Can you work these out from the model? Positions are in its coordinate system, mm. A direction names the side the tool comes from. Coordinates: 2 decimals unless noted, no trailing zeros. Order: outer loops, then holes, each group sorted by start corner. A loop starts at its lowest first (then second) coordinate and runs counter-clockwise, first axis right, second up. Notation, with made-up numbers: (63.5, 5) - (67.5, 5) arc R29 ccw to (67.5, 29) - close; hole circle Ø2 at (20, 35). An arc over 180 degrees is marked (long way). Return JSON: item names as keys, results as strings. Group by question number.
1) Imagine slicing it at C-C (z = -1). Give the number of separate pieces and of enclosed holes in the cut face, and give its area (3 significant figures).
2) Which directions (+Z, -Z, +X, -X, +Y, -Y) give clear straight access to the entire face, cutting with the end or side of a thin tool? Please do faces 4 (the face through (10.377, 0.493, -16.829)), 5 (the face through (-1.235, -2, -6)), 6 (the face through (13, -2, -14.299)), 7 (the face through (2, 7, -7.799)).
3) Imagine slicing it at A-A (z = 2). Write out the boundary of the cut face in (x, y), and give its area (3 significant figures).
4) Imagine slicing it at D-D (x = -13). Write out the boundary of the cut face in (y, z).
5) For pin 1 Ø1.2 at (x, y) = (12.5, -3) entering from -Z; pin 2 Ø0.8 at (x, y) = (-12, 0.5) entering from +Z; pin 3 Ø4 at (x, z) = (-16.5, -16.5) entering from -Y, each with a flat end and sliding along its axis, tell me the tip position at first contact or that it passes through.
6) Imagine slicing it at B-B (x = 25). Write out the boundary of the cut face in (y, z).
7) If we mould it in two halves opening along X, with no side actions, what happens to faces 1 (the face through (13, -5, -7)), 2 (the face through (21, 1, -16)), 3 (the face through (20.765, -2, -6))? For each: pulls with the +X half, pulls with the -X half, needs draft (parallel to the pull), parting line crosses it, or undercut.
8) If I drill on line 1 along X through (y, z) = (8.75, -5.5); line 2 along X through (y, z) = (3, -16.75); line 3 along Z through (x, y) = (-8, 2.75), over which ranges is the centre line in solid material (lowest first)?
```python
from build123d import *

# Parameters (mm, degrees)
SKETCH1_R           = 3
SKETCH1_R_2         = 1.7
BOSS_EXTRUDE1_DEPTH = 1
SKETCH1_4_W         = 1
SKETCH1_4_H         = 0.5
SKETCH1_4_H_2       = 12.5
SKETCH1_4_W_2       = 1.5
SKETCH1_4_W_3       = 2
SKETCH1_4_R         = 1.7
BOSS_EXTRUDE2_DEPTH = 14
SKETCH1_5_W         = 1
SKETCH1_5_H         = 6
SKETCH1_5_H_2       = 0.5
SKETCH1_5_W_2       = 1.5
BOSS_EXTRUDE3_DEPTH = 5


with BuildPart() as part:
    # Sketch1 → Boss-Extrude1 (new body)
    with BuildSketch(Plane(origin=(0, 0, 0), x_dir=(1, 0, 0), z_dir=(0, 1, 0))):
        Polygon((18.764581115, -4.700712669), (40.514581115, -4.700712669), (40.514581115, 20.799287331), (26.264581115, 20.799287331), (26.264581115, 20.299287331), (21.264581115, 20.299287331), (21.264581115, 20.799287331), (11.264581115, 20.799287331), (11.264581115, 20.299287331), (6.264581115, 20.299287331), (6.264581115, 20.799287331), (1.264581115, 20.799287331), (-2.735418885, 20.799287331), (-2.735418885, 20.299287331), (-7.735418885, 20.299287331), (-7.735418885, 20.799287331), (-29.485418885, 20.799287331), (-29.485418885, -4.700712669), (-14.735418885, -4.700712669), (-14.735418885, -4.200712669), (-9.735418885, -4.200712669), (-9.735418885, -4.700712669), (-4.735418885, -4.700712669), (-0.735418885, -4.700712669), (-0.735418885, -4.200712669), (4.264581115, -4.200712669), (4.264581115, -4.700712669), (13.764581115, -4.700712669), (13.764581115, -4.200712669), (18.764581115, -4.200712669), align=None)
        with Locations((-12.235418885, 1.799287331)):
            Circle(SKETCH1_R, mode=Mode.SUBTRACT)
        with Locations((1.764581115, 1.799287331)):
            Circle(SKETCH1_R, mode=Mode.SUBTRACT)
        with Locations((16.264581115, 1.799287331)):
            Circle(SKETCH1_R, mode=Mode.SUBTRACT)
        with Locations((35.389581115, 8.049287331)):
            Circle(SKETCH1_R_2, mode=Mode.SUBTRACT)
        with Locations((-24.110418885, 8.049287331)):
            Circle(SKETCH1_R_2, mode=Mode.SUBTRACT)
        with Locations((-5.235418885, 14.299287331)):
            Circle(SKETCH1_R, mode=Mode.SUBTRACT)
        with Locations((8.764581115, 14.299287331)):
            Circle(SKETCH1_R, mode=Mode.SUBTRACT)
        with Locations((23.764581115, 14.299287331)):
            Circle(SKETCH1_R, mode=Mode.SUBTRACT)
    extrude(amount=BOSS_EXTRUDE1_DEPTH)

    # Sketch1_4 → Boss-Extrude2 (add)
    with BuildSketch(Plane(origin=(0, 0, 0), x_dir=(1, 0, 0), z_dir=(0, 1, 0))):
        Polygon((-18.235418885, -4.200712669), (-18.235418885, 7.799287331), (-11.735418885, 7.799287331), (-11.735418885, 8.299287331), (-18.735418885, 8.299287331), (-18.735418885, -4.700712669), (-14.735418885, -4.700712669), (-14.735418885, -4.200712669), align=None)
        Polygon((-11.735418885, 20.799287331), (-11.735418885, 8.299287331), (-11.235418885, 8.299287331), (-11.235418885, 20.299287331), (-7.735418885, 20.299287331), (-7.735418885, 20.799287331), align=None)
        Polygon((-11.735418885, 8.299287331), (-11.735418885, 7.799287331), (-9.235418885, 7.799287331), (-9.235418885, 8.299287331), (-11.235418885, 8.299287331), align=None)
        Polygon((-6.235418885, -4.200712669), (-9.735418885, -4.200712669), (-9.735418885, -4.700712669), (-5.735418885, -4.700712669), (-5.735418885, 7.799287331), (-6.235418885, 7.799287331), align=None)
        with Locations((-8.735418885, 8.049287331)):
            Rectangle(SKETCH1_4_W, SKETCH1_4_H)
        Polygon((-8.235418885, 8.299287331), (-8.235418885, 7.799287331), (-6.235418885, 7.799287331), (-5.735418885, 7.799287331), (-5.735418885, 8.299287331), align=None)
        with Locations((-5.235418885, 8.049287331)):
            Rectangle(SKETCH1_4_W, SKETCH1_4_H)
        with Locations((-5.235418885, 1.549287331)):
            Rectangle(SKETCH1_4_W, SKETCH1_4_H_2)
        Polygon((-4.735418885, 7.799287331), (-4.735418885, -4.700712669), (-0.735418885, -4.700712669), (-0.735418885, -4.200712669), (-4.235418885, -4.200712669), (-4.235418885, 7.799287331), align=None)
        Polygon((-4.735418885, 8.299287331), (-4.735418885, 7.799287331), (-4.235418885, 7.799287331), (-2.235418885, 7.799287331), (-2.235418885, 8.299287331), align=None)
        with Locations((-1.735418885, 8.049287331)):
            Rectangle(SKETCH1_4_W, SKETCH1_4_H)
        Polygon((0.764581115, 8.299287331), (-1.235418885, 8.299287331), (-1.235418885, 7.799287331), (1.264581115, 7.799287331), (1.264581115, 8.299287331), align=None)
        Polygon((-2.735418885, 20.799287331), (-2.735418885, 20.299287331), (0.764581115, 20.299287331), (0.764581115, 8.299287331), (1.264581115, 8.299287331), (1.264581115, 20.799287331), align=None)
        with Locations((1.764581115, 14.549287331)):
            Rectangle(SKETCH1_4_W, SKETCH1_4_H_2)
        with Locations((1.764581115, 8.049287331)):
            Rectangle(SKETCH1_4_W, SKETCH1_4_H)
        Polygon((6.264581115, 20.799287331), (2.264581115, 20.799287331), (2.264581115, 8.299287331), (2.764581115, 8.299287331), (2.764581115, 20.299287331), (6.264581115, 20.299287331), align=None)
        Polygon((2.764581115, 8.299287331), (2.264581115, 8.299287331), (2.264581115, 7.799287331), (4.764581115, 7.799287331), (4.764581115, 8.299287331), align=None)
        with Locations((5.264581115, 8.049287331)):
            Rectangle(SKETCH1_4_W, SKETCH1_4_H)
        Polygon((5.764581115, 7.799287331), (7.764581115, 7.799287331), (8.264581115, 7.799287331), (8.264581115, 8.299287331), (5.764581115, 8.299287331), align=None)
        Polygon((7.764581115, -4.200712669), (4.264581115, -4.200712669), (4.264581115, -4.700712669), (8.264581115, -4.700712669), (8.264581115, 7.799287331), (7.764581115, 7.799287331), align=None)
        with Locations((9.014581115, 8.049287331)):
            Rectangle(SKETCH1_4_W_2, SKETCH1_4_H)
        Polygon((9.764581115, 8.299287331), (9.764581115, 7.799287331), (10.264581115, 7.799287331), (11.764581115, 7.799287331), (11.764581115, 8.299287331), align=None)
        with Locations((9.014581115, 1.549287331)):
            Rectangle(SKETCH1_4_W_2, SKETCH1_4_H_2)
        Polygon((9.764581115, 7.799287331), (9.764581115, -4.700712669), (13.764581115, -4.700712669), (13.764581115, -4.200712669), (10.264581115, -4.200712669), (10.264581115, 7.799287331), align=None)
        with Locations((12.514581115, 8.049287331)):
            Rectangle(SKETCH1_4_W_2, SKETCH1_4_H)
        Polygon((15.264581115, 8.299287331), (14.764581115, 8.299287331), (13.264581115, 8.299287331), (13.264581115, 7.799287331), (15.264581115, 7.799287331), align=None)
        Polygon((11.264581115, 20.799287331), (11.264581115, 20.299287331), (14.764581115, 20.299287331), (14.764581115, 8.299287331), (15.264581115, 8.299287331), (15.264581115, 20.799287331), align=None)
        with Locations((16.264581115, 8.049287331)):
            Rectangle(SKETCH1_4_W_3, SKETCH1_4_H)
        Polygon((17.764581115, 8.299287331), (17.264581115, 8.299287331), (17.264581115, 7.799287331), (19.264581115, 7.799287331), (19.264581115, 8.299287331), align=None)
        Polygon((19.264581115, 20.799287331), (17.264581115, 20.799287331), (17.264581115, 8.299287331), (17.764581115, 8.299287331), (17.764581115, 20.299287331), (21.264581115, 20.299287331), (21.264581115, 20.799287331), (20.764581115, 20.799287331), align=None)
        with Locations((20.014581115, 8.049287331)):
            Rectangle(SKETCH1_4_W_2, SKETCH1_4_H)
        Polygon((20.764581115, 7.799287331), (22.264581115, 7.799287331), (22.764581115, 7.799287331), (22.764581115, 8.299287331), (20.764581115, 8.299287331), align=None)
        Polygon((22.264581115, -4.200712669), (18.764581115, -4.200712669), (18.764581115, -4.700712669), (19.264581115, -4.700712669), (20.764581115, -4.700712669), (22.764581115, -4.700712669), (22.764581115, 7.799287331), (22.264581115, 7.799287331), align=None)
        Polygon((22.764581115, 8.299287331), (22.764581115, 7.799287331), (30.264581115, 7.799287331), (30.264581115, 20.799287331), (26.264581115, 20.799287331), (26.264581115, 20.299287331), (29.764581115, 20.299287331), (29.764581115, 8.299287331), align=None)
        Polygon((30.264581115, 7.799287331), (22.764581115, 7.799287331), (22.764581115, -4.700712669), (40.514581115, -4.700712669), (40.514581115, 20.799287331), (30.264581115, 20.799287331), align=None)
        with Locations((35.389581115, 8.049287331)):
            Circle(SKETCH1_4_R, mode=Mode.SUBTRACT)
        Polygon((-18.735418885, 8.299287331), (-11.735418885, 8.299287331), (-11.735418885, 20.799287331), (-29.485418885, 20.799287331), (-29.485418885, -4.700712669), (-18.735418885, -4.700712669), align=None)
        with Locations((-24.110418885, 8.049287331)):
            Circle(SKETCH1_4_R, mode=Mode.SUBTRACT)
        with Locations((16.264581115, 14.549287331)):
            Rectangle(SKETCH1_4_W_3, SKETCH1_4_H_2)
    extrude(amount=BOSS_EXTRUDE2_DEPTH)

    # Sketch1_5 → Boss-Extrude3 (add)
    with BuildSketch(Plane(origin=(0, 0, 0), x_dir=(1, 0, 0), z_dir=(0, 1, 0))):
        with Locations((-8.735418885, 11.299287331)):
            Rectangle(SKETCH1_5_W, SKETCH1_5_H)
        Polygon((-8.235418885, 7.799287331), (-9.235418885, 7.799287331), (-9.235418885, 1.799287331), (-9.235418885, -1.200712669), (-8.235418885, -1.200712669), align=None)
        with Locations((-8.735418885, 8.049287331)):
            Rectangle(SKETCH1_5_W, SKETCH1_5_H_2)
        Polygon((-1.235418885, 7.799287331), (-2.235418885, 7.799287331), (-2.235418885, -1.200712669), (-1.235418885, -1.200712669), (-1.235418885, 1.799287331), align=None)
        with Locations((-1.735418885, 11.299287331)):
            Rectangle(SKETCH1_5_W, SKETCH1_5_H)
        with Locations((-1.735418885, 8.049287331)):
            Rectangle(SKETCH1_5_W, SKETCH1_5_H_2)
        Polygon((4.764581115, 7.799287331), (4.764581115, 1.799287331), (4.764581115, -1.200712669), (5.764581115, -1.200712669), (5.764581115, 7.799287331), align=None)
        with Locations((5.264581115, 11.299287331)):
            Rectangle(SKETCH1_5_W, SKETCH1_5_H)
        with Locations((5.264581115, 8.049287331)):
            Rectangle(SKETCH1_5_W, SKETCH1_5_H_2)
        with Locations((12.514581115, 11.299287331)):
            Rectangle(SKETCH1_5_W_2, SKETCH1_5_H)
        with Locations((12.514581115, 8.049287331)):
            Rectangle(SKETCH1_5_W_2, SKETCH1_5_H_2)
        Polygon((13.264581115, 7.799287331), (11.764581115, 7.799287331), (11.764581115, -1.200712669), (13.264581115, -1.200712669), (13.264581115, 1.799287331), align=None)
        Polygon((19.264581115, 7.799287331), (19.264581115, 1.799287331), (19.264581115, -1.200712669), (20.764581115, -1.200712669), (20.764581115, 7.799287331), align=None)
        with Locations((20.014581115, 8.049287331)):
            Rectangle(SKETCH1_5_W_2, SKETCH1_5_H_2)
        with Locations((20.014581115, 11.299287331)):
            Rectangle(SKETCH1_5_W_2, SKETCH1_5_H)
    extrude(amount=-BOSS_EXTRUDE3_DEPTH)


solid = part.part
```
Calculated:
{
 "1": {"separate pieces": "4", "enclosed holes": "0", "area": "525 mm2"},
 "2": {"face 4": "+Y, -Y", "face 5": "+Z, -Z, -Y", "face 6": "-Z, +X, -X, -Y", "face 7": "+Y"},
 "3": {"outline": "(-29.49, 0) - (40.51, 0) - (40.51, 14) - (22.26, 14) - (22.26, 1) - (10.26, 1) - (10.26, 14) - (7.76, 14) - (7.76, 1) - (-4.24, 1) - (-4.24, 14) - (-6.24, 14) - (-6.24, 1) - (-18.24, 1) - (-18.24, 14) - (-29.49, 14) - close", "area": "512 mm2"},
 "4": {"outline": "(0, -20.8) - (14, -20.8) - (14, -7.8) - (1, -7.8) - (1, -4.7) - (0, -4.7) - close; (0, 1.1) - (1, 1.1) - (1, 4.2) - (0, 4.2) - close"},
 "5": {"pin 1": "z = -14.3", "pin 2": "z = 4.2", "pin 3": "y = 0"},
 "6": {"outline": "(0, -20.3) - (1, -20.3) - (1, -17.03) - (0, -17.03) - close; (0, -11.57) - (1, -11.57) - (1, -8.3) - (14, -8.3) - (14, 4.7) - (0, 4.7) - close"},
 "7": {"face 1": "needs draft", "face 2": "undercut", "face 3": "pulls with the +X half"},
 "8": {"line 1": "-29.49 to -18.24, -6.24 to -4.24, 7.76 to 10.26, 22.26 to 40.51", "line 2": "-29.49 to -11.24, 0.76 to 2.76, 14.76 to 17.76, 29.76 to 40.51", "line 3": "-20.8 to -20.3, -8.3 to -7.8, 4.2 to 4.7"}
}
